Geometry check sheet. Reference: the model listing, model coordinates, mm. Round coordinates to 2 decimals unless told otherwise and drop trailing zeros. Order: outer loops, then holes, each group sorted by start corner. A loop starts at its lowest first (then second) coordinate and runs counter-clockwise, first axis right, second up. Notation, with made-up numbers: M 29,-9 L 75,-9 A18 cw 75,24 Z; hole C -24.5,-16 d8. An arc over 180 degrees is marked long. Return JSON: item names as keys, results as strings. Group by question number.
```python
from build123d import *

# Parameters (mm, degrees)
F0_R     = 23.5
F0_R_2   = 10
F1_DEPTH = 7
F2_R     = 0.5


with BuildPart() as f1:
    # F0 (on Top) → F1 (new body, symmetric)
    with BuildSketch(Plane.XY):
        Circle(F0_R)
        Circle(F0_R_2, mode=Mode.SUBTRACT)
    extrude(amount=F1_DEPTH, both=True)

    # F2
    f2_edges = [f1.edges().sort_by_distance(p)[0] for p in [
        (-23.5, 0, -7),
        (23.5, 0, 0),
        (-23.5, 0, 7),
        (-10, 0, 7),
        (10, 0, 0),
        (-10, 0, -7),
    ]]
    fillet(f2_edges, radius=F2_R)


solid = f1.part
```
Q1. Section check C-C on z = 2.75. Record the cut outline in (x, y).
Q2. Section check A-A on y = 0. Record the cut outline in (x, z).
Q3. Material ranges on line 1 along Y through (x, z) = (0, -1); line 2 along Y through (x, z) = (-5, -1.5); line 3 along X through (y, z) = (8.5, 1.75), recorded low to high.
Q4. Release check for a two-part mould opening along X. For faces 1 (the face through (-2.17, -9.76, -0.09)), 2 (the face through (10, -5, -7)), 3 (the face through (22.4, 7.1, 0.1)) record: +X half, -X half, draft (parallel to the pull), parting line (faces both ways), or undercut.
Q5. Depth check by flat-ended pin: pin 1 Ø3 at (x, z) = (4.5, 3) entering from +Y; pin 2 Ø4 at (y, z) = (3, -5) entering from +X; pin 3 Ø4 at (y, z) = (11, -5.5) entering from +X. Enter the tip coordinate at first touch or a pass-through.
Geometry check:
{
 "1": {"outline": "C 0,0 d47; hole C 0,0 d20"},
 "2": {"outline": "M -23.5,-6.5 A0.5 ccw -23,-7 L -10.5,-7 A0.5 ccw -10,-6.5 L -10,6.5 A0.5 ccw -10.5,7 L -23,7 A0.5 ccw -23.5,6.5 Z; M 10,-6.5 A0.5 ccw 10.5,-7 L 23,-7 A0.5 ccw 23.5,-6.5 L 23.5,6.5 A0.5 ccw 23,7 L 10.5,7 A0.5 ccw 10,6.5 Z"},
 "3": {"line 1": "y = -23.5 to -10, 10 to 23.5", "line 2": "y = -22.96 to -8.66, 8.66 to 22.96", "line 3": "x = -21.91 to -5.27, 5.27 to 21.91"},
 "4": {"face 1": "undercut", "face 2": "draft", "face 3": "parting line"},
 "5": {"pin 1": "stops at y = 23.31", "pin 2": "stops at x = 23.48", "pin 3": "stops at x = 21.71"}
}
